Here's how the part is built. I have some questions about the finished solid (model axes, mm). Face numbers are marked on the shaded views. A direction names the side the tool comes from. Coordinates: 2 decimals unless noted, no trailing zeros. Loops run counter-clockwise (first coordinate to the right, second up) from the corner with the lowest first, then second, coordinate; pieces in that order, holes last. Notation, with made-up numbers: M -33.75,64.5 L -9.75,64.5 A12 cw -9.75,83.5 Z; hole C 56,80.5 d1. An arc over 180 degrees is marked long. Use one line per item in the form item = value. Start each with the question number.
(1) On a 3-axis mill with a long thin cutter (end or side, diameter ignored), from which of +Z, -Z, +X, -X, +Y, -Y can I reach the whole of each face in a straight line? I mean the marked faces 1 and 2. Say none if no direction works.
(2) Please list where these lines run through material, in increasing order: L1, parallel to Z at x = -8, y = -4; L2, parallel to Z at x = -12, y = 11.5; L3, parallel to X at y = -4.5, z = 12.
(3) Imagine slicing it at C-C, the plane x = -25.5. Please give me the cut outline in (y, z).
(4) Thinking about a two-plate mould opening in Z: for the marked faces 3 and 4, which applies, +Z half, -Z half, draft (parallel to the pull), parting line (faces both ways), or undercut?
(5) Imagine slicing it at B-B, the plane x = 24.5. Please give me the cut outline in (y, z) (3 decimals), and give its area (3 significant figures).
(6) Imagine slicing it at A-A, the plane y = 23. Please give me the cut outline in (x, z), and give its area (3 significant figures).
(7) Imagine slicing it at D-D, the plane z = 336. Please give me the cut outline in (x, y), and give its area (3 significant figures).
(8) Will these pins go through, and if not, where does the flat tip stop? P1, Ø10, axis at y = 18.5, z = 157, coming from the +X side; P2, Ø2, axis at x = 2.5, y = 26.5, coming from the +Z side; P3, Ø1, axis at x = 15, y = -14, coming from the -Z side; P4, Ø21, axis at x = -9, y = 12, coming from the +Z side.
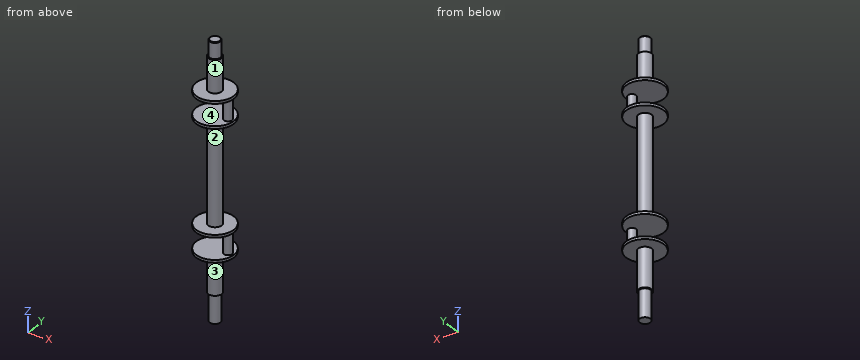
Autodesk Inventor part; units mm, degrees
ref_plane "YZ Plane" through (0, 0, 0) normal (1, 0, 0) x (0, 1, 0)
ref_plane "XZ Plane" through (0, 0, 0) normal (0, 1, 0) x (-1, 0, 0)
ref_plane "XY Plane" through (0, 0, 0) normal (0, 0, 1) x (1, 0, 0)
sketch "草图1" plane through (0, 0, 0) normal (0, 0, 1) x (1, 0, 0)
  circle A0 centre (0, 0) radius 12.5
  dimension "d0" = 25
extrude "拉伸1" add sketch "草图1" along normal blind 103
sketch "草图2" plane through (0, 0, 103) normal (0, 0, 1) x (1, 0, 0)
  circle A0 centre (0, 0) radius 35
  dimension "d3" = 70
extrude "拉伸2" add sketch "草图2" along normal blind 5
sketch "草图3" plane through (0, 0, 108) normal (0, 0, 1) x (1, 0, 0)
  circle A0 centre (24, 0) radius 7.5
  line L0 (0, 0) -> (4.085, 0)
  dimension "d6" = 15
  dimension "d7" = 4.085
  dimension "d8" = 24
extrude "拉伸3" add sketch "草图3" along normal blind 40
sketch "草图4" plane through (24, 0, 148) normal (0, 0, 1) x (1, 0, 0)
  circle A0 centre (-24, 0) radius 35
  circle A1 centre (-24, 0) radius 35
  dimension "d11" = 70
extrude "拉伸4" add sketch "草图4" along normal blind 5
sketch "草图5" plane through (0, 0, 153) normal (0, 0, 1) x (1, 0, 0)
  circle A0 centre (0, 0) radius 12.5
  dimension "d14" = 25
extrude "拉伸5" add sketch "草图5" along normal blind 190
sketch "草图6" plane through (0, 0, 343) normal (0, 0, 1) x (1, 0, 0)
  circle A0 centre (0, 0) radius 35
  dimension "d17" = 70
extrude "拉伸6" add sketch "草图6" along normal blind 5
sketch "草图7" plane through (0, 0, 348) normal (0, 0, 1) x (1, 0, 0)
  circle A0 centre (24, 0) radius 7.5
  circle A1 centre (24, 0) radius 7.5
  point P0 (0, 0)
  dimension "d20" = 15
extrude "拉伸7" add sketch "草图7" along normal blind 40
sketch "草图8" plane through (24, 0, 388) normal (0, 0, 1) x (1, 0, 0)
  circle A0 centre (-24, 0) radius 12.5
  circle A1 centre (-24, 0) radius 35
  dimension "d23" = 70
extrude "拉伸8" add sketch "草图8" along normal blind 5 contours A0 | A1
sketch "草图9" plane through (0, 0, 393) normal (0, 0, 1) x (1, 0, 0)
  circle A0 centre (0, 0) radius 12.5
  dimension "d26" = 25
extrude "拉伸9" add sketch "草图9" along normal blind 90
sketch "草图10" plane through (0, 0, 483) normal (0, 0, 1) x (1, 0, 0)
  circle A0 centre (0, 0) radius 10
  circle A1 centre (0, 0) radius 12.5
  dimension "d32" = 20
  dimension "d33" = 25
extrude "拉伸10" cut sketch "草图10" against normal blind 30
chamfer "倒角2" distance 1 angle 45 1 edges at (-10, 0, 483)
sketch "草图11" plane through (0, 0, 0) normal (0, 0, -1) x (-1, 0, 0)
  circle A0 centre (0, 0) radius 10
  circle A1 centre (0, 0) radius 12.5
  dimension "d39" = 20
  dimension "d40" = 25
extrude "拉伸11" cut sketch "草图11" against normal blind 30
sketch "草图12" plane through (0, 0, 0) normal (0, 0, -1) x (-1, 0, 0)
  circle A0 centre (0, 0) radius 10
  dimension "d43" = 20
extrude "拉伸12" add sketch "草图12" along normal blind 22
properties part number "砂轮架带动曲轴"
Answer:
q1.face_1 = +Z
q1.face_2 = none
q2.L1 = -22 to 108, 148 to 348, 388 to 483
q2.L2 = 103 to 108, 148 to 153, 343 to 348, 388 to 393
q2.L3 = -8.93 to 8.93
q3.outline = M -23.97,103 L 23.97,103 L 23.97,108 L -23.97,108 Z; M -23.97,148 L 23.97,148 L 23.97,153 L -23.97,153 Z; M -23.97,343 L 23.97,343 L 23.97,348 L -23.97,348 Z; M -23.97,388 L 23.97,388 L 23.97,393 L -23.97,393 Z
q4.face_3 = draft
q4.face_4 = undercut
q5.outline = M -24.995,103 L 24.995,103 L 24.995,108 L 7.483,108 L 7.483,148 L 24.995,148 L 24.995,153 L -24.995,153 L -24.995,148 L -7.483,148 L -7.483,108 L -24.995,108 Z; M -24.995,343 L 24.995,343 L 24.995,348 L 7.483,348 L 7.483,388 L 24.995,388 L 24.995,393 L -24.995,393 L -24.995,388 L -7.483,388 L -7.483,348 L -24.995,348 Z
q5.area = 2,200 mm²
q6.outline = M -26.38,103 L 26.38,103 L 26.38,108 L -26.38,108 Z; M -26.38,148 L 26.38,148 L 26.38,153 L -26.38,153 Z; M -26.38,343 L 26.38,343 L 26.38,348 L -26.38,348 Z; M -26.38,388 L 26.38,388 L 26.38,393 L -26.38,393 Z
q6.area = 1,060 mm²
q7.outline = C 0,0 d25
q7.area = 491 mm²
q8.P1 = 31.38
q8.P2 = 393
q8.P3 = 103
q8.P4 = 483
